from build123d import *

# Parameters (mm, degrees)
F2_R     = 6
F3_DEPTH = 25


with BuildPart() as f1:
    # F0 (on Front) → F1 (revolve)
    with BuildSketch(Plane.XZ):
        with BuildLine():
            Line((0, 0), (0, 11))
            Line((0, 11), (-7.851503, 11))
            Line((-7.851503, 11), (-12.61, 8.781077))
            ThreePointArc((-12.61, 8.781077), (-13.228536, 8.571112), (-13.877855, 8.5))
            Line((-13.877855, 8.5), (-20.57, 8.5))
            Line((-20.57, 8.5), (-21.5, 14.5))
            Line((-21.5, 14.5), (-30.571486, 14.5))
            Line((-30.571486, 14.5), (-48.773584, 14.5))
            Line((-48.773584, 14.5), (-48.773584, 11))
            Line((-48.773584, 11), (-53.754714, 11))
            Line((-53.754714, 11), (-53.754714, 14.5))
            Line((-53.754714, 14.5), (-63.094336, 14.5))
            Line((-63.094336, 14.5), (-63.094336, 0))
            Line((-63.094336, 0), (0, 0))
        make_face()
    revolve(axis=Axis((-31.547168, 0, 0), (1, 0, 0)))

    # F2 (on face) → F3 (join)
    with BuildSketch(Plane.YZ):
        Circle(F2_R)
    extrude(amount=-F3_DEPTH)


solid = f1.part
Verification items for the finished model (mm, model axes). A direction names the side the tool comes from. Round coordinates to 2 decimals unless told otherwise and drop trailing zeros. Order: outer loops, then holes, each group sorted by start corner. A loop starts at its lowest first (then second) coordinate and runs counter-clockwise, first axis right, second up. Notation, with made-up numbers: (29.25, 3) -> (72.25, 3) arc R14 ccw to (72.25, 25) -> close; hole circle Ø1 at (42.25, 75). An arc over 180 degrees is marked (long way). Put each result on its own line as item: value.
1) Material ranges on line 1 (X direction, y = -0.5, z = -11.25); line 2 (X direction, y = 2.5, z = 10); line 3 (Z direction, x = -54, y = 2), recorded low to high.
Final values:
line 1: x = -63.09 to -53.75, -48.77 to -21
line 2: x = -63.09 to -20.85, -9.34 to 0
line 3: z = -14.36 to 14.36
2) Section check D-D (x = -28). Record the cut outline in (y, z), then the cut area to 3 significant figures.
Final values:
outline: circle Ø29 at (0, 0)
area: 661 mm^2
3) Mould release check, pull along X, two halves, no side actions. Record for faces 1 (the flat face through (-53.755, -11, 2)), 2 (the flat face through (-63.094, 0, 0)), 3 (the flat face through (0, 0, 0)), 4 (the cylindrical face through (-35.328, 12.864, 6.691)): +X half, -X half, draft (parallel to the pull), parting line (faces both ways), or undercut.
Final values:
face 1: undercut
face 2: -X half
face 3: +X half
face 4: draft
4) Depth check by flat-ended pin: pin 1 (2 mm diameter, centred on x = -21, z = -6.5, fed in from -Y); pin 2 (6 mm diameter, centred on y = 2, z = -0.5, fed in from +X); pin 3 (8 mm diameter, centred on x = -55.5, z = 9, fed in from +Y); pin 4 (6 mm diameter, centred on x = -47.5, z = -8.5, fed in from +Y). Enter the tip coordinate at first touch or a pass-through.
Final values:
pin 1: stops at y = -13.36
pin 2: stops at x = 0
pin 3: stops at y = 13.61
pin 4: stops at y = 13.42
5) Section check C-C (x = -52). Record the cut outline in (y, z), then the cut area to 3 significant figures.
Final values:
outline: circle Ø22 at (0, 0)
area: 380 mm^2
6) Set-up check for faces 5 (the cylindrical face through (-58.49, 12.864, 6.691)), 6 (the cylindrical face through (-3.98, 10.74, -2.38)), 7 (the conical face through (-12.38, 5.41, -7.05)): record each of +Z, -Z, +X, -X, +Y, -Y from which the full face is reachable in a straight line by a thin tool's end or side.
Final values:
face 5: +X, -X
face 6: +X
face 7: none
7) Section check A-A (y = 0). Record the cut outline in (x, z).
Final values:
outline: (-63.09, -14.5) -> (-53.75, -14.5) -> (-53.75, -11) -> (-48.77, -11) -> (-48.77, -14.5) -> (-21.5, -14.5) -> (-20.57, -8.5) -> (-13.88, -8.5) arc R3 cw to (-12.61, -8.78) -> (-7.85, -11) -> (0, -11) -> (0, 11) -> (-7.85, 11) -> (-12.61, 8.78) arc R3 cw to (-13.88, 8.5) -> (-20.57, 8.5) -> (-21.5, 14.5) -> (-48.77, 14.5) -> (-48.77, 11) -> (-53.75, 11) -> (-53.75, 14.5) -> (-63.09, 14.5) -> close
